Geometry: final body of the model. Coordinates: model frame, mm. Face numbers are marked on the shaded views. A direction names the side the tool comes from. Give positions to 0.01 mm unless a question says otherwise; leave off trailing zeros. Write each loop counter-clockwise with the first axis right and the second up, starting at its lowest first coordinate (ties: lowest second). Pieces come first, ordered by that corner, then holes. Notation, with made-up numbers: M -11.5,59.25 L 12.5,59.25 A22 cw 12.5,68.25 Z; hole C -24,6.5 d5. An arc over 180 degrees is marked long. Answer as a JSON object with one key per item and string values.
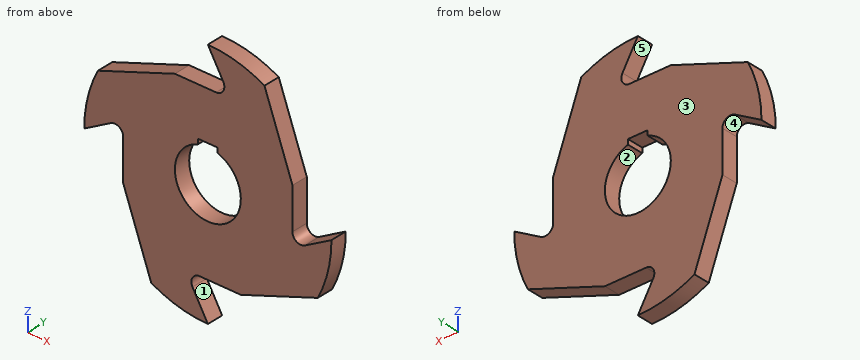
from build123d import *

# Parameters (mm, degrees)
F1_DEPTH = 10


with BuildPart() as f1:
    # F0 (on Front) → F1 (new body)
    with BuildSketch(Plane.XZ):
        with BuildLine():
            Line((-20, 51.339746), (-66.669677, 34.353373))
            ThreePointArc((-66.669677, 34.353373), (-72.887673, 17.674477), (-75, 0))
            Line((-75, 0), (-58.839746, 9.330127))
            ThreePointArc((-58.839746, 9.330127), (-53.839746, 9.330127), (-51.339746, 5))
            Line((-51.339746, 5), (-51.339746, -20))
            Line((-51.339746, -20), (-34.353373, -66.669677))
            ThreePointArc((-34.353373, -66.669677), (-17.674477, -72.887673), (0, -75))
            Line((0, -75), (-9.330127, -58.839746))
            ThreePointArc((-9.330127, -58.839746), (-9.330127, -53.839746), (-5, -51.339746))
            Line((-5, -51.339746), (20, -51.339746))
            Line((20, -51.339746), (66.669677, -34.353373))
            ThreePointArc((66.669677, -34.353373), (72.887673, -17.674477), (75, 0))
            Line((75, 0), (58.839746, -9.330127))
            ThreePointArc((58.839746, -9.330127), (53.839746, -9.330127), (51.339746, -5))
            Line((51.339746, -5), (51.339746, 20))
            Line((51.339746, 20), (34.353373, 66.669677))
            ThreePointArc((34.353373, 66.669677), (17.674477, 72.887673), (0, 75))
            Line((0, 75), (9.330127, 58.839746))
            ThreePointArc((9.330127, 58.839746), (9.330127, 53.839746), (5, 51.339746))
            Line((5, 51.339746), (0, 51.339746))
            Line((0, 51.339746), (-20, 51.339746))
        make_face()
        with BuildLine():
            Line((-6, 22.078784), (0, 22.078784))
            Line((0, 22.078784), (6, 22.078784))
            Line((6, 22.078784), (6, 19.078784))
            ThreePointArc((6, 19.078784), (0, -20), (-6, 19.078784))
            Line((-6, 19.078784), (-6, 22.078784))
        make_face(mode=Mode.SUBTRACT)
    extrude(amount=F1_DEPTH)


solid = f1.part
1) Pull-direction query (X, two-part tool) for the marked faces 1, 2 and 3; classes: pulls with the +X half, pulls with the -X half, needs draft (parallel to the pull), parting line crosses it, or undercut.
Geometry check:
{"face 1": "pulls with the +X half", "face 2": "undercut", "face 3": "needs draft"}
2) Contact query for flat-ended pins moving along their axis: P1, Ø2.5, axis at y = -4, z = 20, coming from the +X side; P2, Ø5, axis at x = -11, z = -12.5, coming from the +Y side; P3, Ø3.5, axis at y = -4, z = 20.5, coming from the -X side; P4, Ø3, axis at x = -4.5, y = -4.5, coming from the +Z side. Output: stop coordinate, or through.
Geometry check:
{"P1": "stops at x = 51.34", "P2": "passes through", "P3": "stops at x = -72.62", "P4": "stops at z = 51.34"}
3) Line query: line 1 (Z direction, x = 3.5, y = -9); line 2 (X direction, y = -9, z = 18); line 3 (Z direction, x = 7, y = -2.5) (3 decimals). Output: solid intervals per line, ascending. Write a range as from..to.
Geometry check:
{"line 1": "z = -51.34..-19.69, 22.08..51.34, 68.94..74.92", "line 2": "x = -72.81..-8.72, 8.72..51.34", "line 3": "z = -51.34..-18.735, 18.735..51.757, 62.876..74.673"}
4) Cut plane B-B on z = -28. Return loops of the section in (x, y).
Geometry check:
{"outline": "M -48.43,-10 L 69.58,-10 L 69.58,0 L -48.43,0 Z"}
5) Cut plane C-C on x = 62. Return loops of the section in (y, z), and give its area (3 significant figures).
Geometry check:
{"outline": "M -10,-36.05 L 0,-36.05 L 0,-7.51 L -10,-7.51 Z", "area": "285 mm2"}
6) Cut plane A-A on y = -3.25. Return loops of the section in (x, z).
Geometry check:
{"outline": "M -75,0 L -58.84,9.33 A5 cw -51.34,5 L -51.34,-20 L -34.35,-66.67 A75 ccw 0,-75 L -9.33,-58.84 A5 cw -5,-51.34 L 20,-51.34 L 66.67,-34.35 A75 ccw 75,0 L 58.84,-9.33 A5 cw 51.34,-5 L 51.34,20 L 34.35,66.67 A75 ccw 0,75 L 9.33,58.84 A5 cw 5,51.34 L -20,51.34 L -66.67,34.35 A75 ccw Z; hole M -6,19.08 A20 ccw long 6,19.08 L 6,22.08 L -6,22.08 Z"}
7) Set-up query: the marked faces 4 and 5. Return all of +Z, -Z, +X, -X, +Y, -Y with unobstructed straight access to the full face (end or side cutting, diameter ignored); none if empty.
Geometry check:
{"face 4": "-Z, +Y, -Y", "face 5": "-X, +Y, -Y"}
